Work out the finished part from the listing and answer in its coordinate system (mm). A direction names the side the tool comes from. Coordinates: 2 decimals unless noted, no trailing zeros. Loops run counter-clockwise (first coordinate to the right, second up) from the corner with the lowest first, then second, coordinate; pieces in that order, holes last. Notation, with made-up numbers: (80, 25) - (101, 25) arc R25 ccw to (101, 38) - close; hole circle Ø5 at (-25, 46.25). An arc over 180 degrees is marked (long way). Write each question's results on one line, items separated by ' | '. Start each with the question number.
1. Find the intervals of material crossed by line 1 along X through (y, z) = (-0.2, 4.5); line 2 along Z through (x, y) = (-2.75, 1.95); line 3 along Y through (x, z) = (0.5, 4.25), in increasing order. Write a range as [from, to].
2. A cutting plane is placed at C-C on x = 0.25. Determine the outline of the cut face in (y, z), then the cut area to 3 significant figures.
3. Which of the six approach directions +Z, -Z, +X, -X, +Y, -Y give full straight-line access (tool end or side, diameter ignored) to faces 1 (the flat face through (0, 1.75, 5)), 2 (the flat face through (0, -1.75, 5)), 3 (the flat face through (0, -2, 3))?
4. A cutting plane is placed at A-A on y = 0.8. Determine the outline of the cut face in (x, z).
5. Each of these flat-tipped pins is pushed along its axis until it touches: P1, Ø1.5, axis at x = -2.5, y = 1.5, coming from the -Z side; P2, Ø1.8, axis at x = 1, z = 4.5, coming from the +Y side; P3, Ø1.8, axis at x = -1, z = 4.5, coming from the -Y side; P4, Ø1.2, axis at y = 0, z = 4.5, coming from the +X side. Where does it stop, or does it pass through?
6. A cutting plane is placed at B-B on z = 5.75. Determine the outline of the cut face in (x, y).
7. A cutting plane is placed at D-D on z = 6.75. Determine the outline of the cut face in (x, y), then the cut area to 3 significant figures.
from build123d import *

# Parameters (mm, degrees)
SKETCH_1_W      = 7
SKETCH_1_H      = 5
EXTRUDE_1_DEPTH = 3
SKETCH_2_W      = 5.5
SKETCH_2_H      = 3.5
EXTRUDE_2_DEPTH = 4
FILLET_1_R      = 0.5
FILLET_2_R      = 0.5


with BuildPart() as part:
    # 草图1 → 凸台-拉伸1 (new body)
    with BuildSketch(Plane.XY):
        Rectangle(SKETCH_1_W, SKETCH_1_H)
    extrude(amount=EXTRUDE_1_DEPTH)

    # 草图2 → 凸台-拉伸2 (add)
    with BuildSketch(Plane.XY.offset(3)):
        Rectangle(SKETCH_2_W, SKETCH_2_H)
    extrude(amount=EXTRUDE_2_DEPTH)

    # 圆角1
    fillet_1_edges = [part.edges().sort_by_distance(p)[0] for p in [
        (2.75, 0, 7),
        (0, 1.75, 7),
        (-2.75, 0, 7),
        (0, -1.75, 7),
    ]]
    fillet(fillet_1_edges, radius=FILLET_1_R)

    # 圆角2
    # the kernel refuses this fillet: 0.5 mm, written as the material it takes off along each edge
    with BuildSketch(Plane(origin=(-2.25, 1.25, 6.5), x_dir=(-1, 0, 0), z_dir=(0, 1, 0))) as fillet_2_piece_1_section:
        Polygon((0, 0), (FILLET_2_R, 0), (FILLET_2_R, FILLET_2_R), (0, FILLET_2_R), align=None)
    fillet_2_piece_1 = extrude(amount=FILLET_2_R, mode=Mode.PRIVATE)
    fillet_2_piece_1 = fillet_2_piece_1 - Plane(origin=(-2.25, 1.25, 6.5), x_dir=(0.7071067811865475, 0, -0.7071067811865475), z_dir=(0, 1, 0)) * Sphere(FILLET_2_R, mode=Mode.PRIVATE)
    add(fillet_2_piece_1, mode=Mode.SUBTRACT)
    with BuildSketch(Plane(origin=(2.25, 1.25, 6.5), x_dir=(1, 0, 0), z_dir=(0, 1, 0))) as fillet_2_piece_2_section:
        Polygon((0, 0), (FILLET_2_R, 0), (FILLET_2_R, -FILLET_2_R), (0, -FILLET_2_R), align=None)
    fillet_2_piece_2 = extrude(amount=FILLET_2_R, mode=Mode.PRIVATE)
    fillet_2_piece_2 = fillet_2_piece_2 - Plane(origin=(2.25, 1.25, 6.5), x_dir=(-0.7071067811865475, 0, -0.7071067811865475), z_dir=(0, 1, 0)) * Sphere(FILLET_2_R, mode=Mode.PRIVATE)
    add(fillet_2_piece_2, mode=Mode.SUBTRACT)
    with BuildSketch(Plane(origin=(-2.25, -1.25, 6.5), x_dir=(0, -1, 0), z_dir=(-1, 0, 0))) as fillet_2_piece_3_section:
        Polygon((0, 0), (FILLET_2_R, 0), (FILLET_2_R, FILLET_2_R), (0, FILLET_2_R), align=None)
    fillet_2_piece_3 = extrude(amount=FILLET_2_R, mode=Mode.PRIVATE)
    fillet_2_piece_3 = fillet_2_piece_3 - Plane(origin=(-2.25, -1.25, 6.5), x_dir=(0, 0.7071067811865475, -0.7071067811865475), z_dir=(-1, 0, 0)) * Sphere(FILLET_2_R, mode=Mode.PRIVATE)
    add(fillet_2_piece_3, mode=Mode.SUBTRACT)
    with BuildSketch(Plane(origin=(2.25, -1.25, 6.5), x_dir=(0, -1, 0), z_dir=(1, 0, 0))) as fillet_2_piece_4_section:
        Polygon((0, 0), (FILLET_2_R, 0), (FILLET_2_R, -FILLET_2_R), (0, -FILLET_2_R), align=None)
    fillet_2_piece_4 = extrude(amount=FILLET_2_R, mode=Mode.PRIVATE)
    fillet_2_piece_4 = fillet_2_piece_4 - Plane(origin=(2.25, -1.25, 6.5), x_dir=(0, 0.7071067811865475, -0.7071067811865475), z_dir=(1, 0, 0)) * Sphere(FILLET_2_R, mode=Mode.PRIVATE)
    add(fillet_2_piece_4, mode=Mode.SUBTRACT)
    with BuildSketch(Plane(origin=(2.75, -1.75, 3), x_dir=(0, 1, 0), z_dir=(0, 0, 1)), Plane(origin=(2.75, 1.75, 3), x_dir=(-1, 0, 0), z_dir=(0, 0, 1))) as fillet_2_piece_5:
        with BuildLine():
            CenterArc((FILLET_2_R, FILLET_2_R), FILLET_2_R, 180, 90)
            Line((0, FILLET_2_R), (0, 0))
            Line((0, 0), (FILLET_2_R, 0))
        make_face()
    extrude(amount=3.5, mode=Mode.SUBTRACT)
    with BuildSketch(Plane(origin=(-2.75, -1.75, 3), x_dir=(0, 1, 0), z_dir=(0, 0, 1)), Plane(origin=(-2.75, 1.75, 3), x_dir=(1, 0, 0), z_dir=(0, 0, 1))) as fillet_2_piece_6:
        with BuildLine():
            CenterArc((FILLET_2_R, -FILLET_2_R), FILLET_2_R, 90, 90)
            Line((0, -FILLET_2_R), (0, 0))
            Line((0, 0), (FILLET_2_R, 0))
        make_face()
    extrude(amount=3.5, mode=Mode.SUBTRACT)


solid = part.part
Values:
1) line 1: [-2.75, 2.75] | line 2: [0, 3] | line 3: [-1.75, 1.75]
2) outline: (-2.5, 0) - (2.5, 0) - (2.5, 3) - (1.75, 3) - (1.75, 6.5) arc R0.5 ccw to (1.25, 7) - (-1.25, 7) arc R0.5 ccw to (-1.75, 6.5) - (-1.75, 3) - (-2.5, 3) - close | area: 28.9 mm^2
3) face 1: +Z, +X, -X, +Y | face 2: +Z, +X, -X, -Y | face 3: +Z
4) outline: (-3.5, 0) - (3.5, 0) - (3.5, 3) - (2.75, 3) - (2.75, 6.5) arc R0.5 ccw to (2.25, 7) - (-2.25, 7) arc R0.5 ccw to (-2.75, 6.5) - (-2.75, 3) - (-3.5, 3) - close
5) P1: z = 0 | P2: y = 1.75 | P3: y = -1.75 | P4: x = 2.75
6) outline: (-2.75, -1.25) arc R0.5 ccw to (-2.25, -1.75) - (2.25, -1.75) arc R0.5 ccw to (2.75, -1.25) - (2.75, 1.25) arc R0.5 ccw to (2.25, 1.75) - (-2.25, 1.75) arc R0.5 ccw to (-2.75, 1.25) - close
7) outline: (-2.68, -1.25) arc R0.43 ccw to (-2.25, -1.68) - (2.25, -1.68) arc R0.43 ccw to (2.68, -1.25) - (2.68, 1.25) arc R0.43 ccw to (2.25, 1.68) - (-2.25, 1.68) arc R0.43 ccw to (-2.68, 1.25) - close | area: 17.9 mm^2
